The listing builds one solid part. Answer for the finished solid, in the listing's coordinates (mm). Face numbers are marked on the shaded views. A direction names the side the tool comes from. Coordinates: 2 decimals unless noted, no trailing zeros. Order: outer loops, then holes, each group sorted by start corner. A loop starts at its lowest first (then second) coordinate and runs counter-clockwise, first axis right, second up. Notation, with made-up numbers: (-37, 34) -> (-25, 34) arc R14 ccw to (-25, 52) -> close; hole circle Ø11 at (-25.75, 13). An arc over 180 degrees is marked (long way). Answer in a Markdown table with one row per item.
```python
from build123d import *

# Parameters (mm, degrees)
BASPROSKE_W         = 40
BASPROSKE_H         = 25
TOOTHCUT_DEPTH      = 54.38539126
TEETHCUTS_COUNT     = 23
TEETHCUTS_ANGLE     = 344.347826087
BORSKE_R            = 0.4
BORE_DEPTH          = 50.0000508
CUT_EXTRUDE_1_DEPTH = 54.3731118
SKETCH_2_R          = 1.6
CUT_EXTRUDE_2_DEPTH = 54.3731118
EXTRUDE_1_DEPTH     = 40
SKETCH_5_R          = 1.6
CUT_EXTRUDE_3_DEPTH = 61.166132826
CUT_EXTRUDE_4_DEPTH = 61.571969914
SKETCH_7_W          = 12
SKETCH_7_H          = 22
CUT_EXTRUDE_5_DEPTH = 61.166132826
SKETCH_8_R          = 2.6
CUT_EXTRUDE_6_DEPTH = 61.571969914
SKETCH_10_R         = 1.6
SKETCH_10_W         = 12
SKETCH_10_H         = 22
CUT_EXTRUDE_7_DEPTH = 61.166132826
CUT_EXTRUDE_9_DEPTH = 60.774271549


with BuildPart() as part:
    # BasProSke → Base-Revolve (revolve)
    with BuildSketch(Plane(origin=(0, 0, 0), x_dir=(1, 0, 0), z_dir=(0, 1, 0)), mode=Mode.PRIVATE) as base_revolve_sk:
        with Locations((20, 12.5)):
            Rectangle(BASPROSKE_W, BASPROSKE_H)
    revolve(base_revolve_sk.sketch.rotate(Axis((-10, 0, 0), (1, 0, 0)), 180), axis=Axis((-10, 0, 0), (1, 0, 0)))

    # TooCutSke → ToothCut (cut, through all)
    with BuildSketch(Plane(origin=(0, 0, 0), x_dir=(0, 0, -1), z_dir=(1, 0, 0))):
        with BuildLine():
            ThreePointArc((0.960248578, 20.47649686), (0, 20.499), (-0.960248578, 20.47649686))
            ThreePointArc((-0.960248578, 20.47649686), (-1.62297083, 22.794554384), (-2.865164893, 24.860842208))
            ThreePointArc((-2.865164893, 24.860842208), (0, 25.0254), (2.865164893, 24.860842208))
            ThreePointArc((2.865164893, 24.860842208), (1.62297083, 22.794554384), (0.960248578, 20.47649686))
        make_face()
    toothcut = extrude(amount=TOOTHCUT_DEPTH, mode=Mode.SUBTRACT)

    # TeethCuts: ToothCut ×23 about axis
    teethcuts_axis = Axis((-10, 0, 0), (1, 0, 0))
    for i in range(1, TEETHCUTS_COUNT):
        add(toothcut.rotate(teethcuts_axis, i * TEETHCUTS_ANGLE / (TEETHCUTS_COUNT - 1)), mode=Mode.SUBTRACT)

    # BorSke → Bore (cut, symmetric)
    with BuildSketch(Plane(origin=(0, 0, 0), x_dir=(0, 0, -1), z_dir=(1, 0, 0))):
        with Locations(Location((0, 0, 0), (0, 0, 180))):
            Circle(BORSKE_R)
    extrude(amount=BORE_DEPTH, both=True, mode=Mode.SUBTRACT)

    # 草图1 → 切除-拉伸1 (cut, through all)
    with BuildSketch(Plane(origin=(40, 0, 0), x_dir=(0, 0, -1), z_dir=(1, 0, 0))):
        Polygon((0, 0), (0, -25), (-13.134994366, -31.325673685), (-39.860156169, 4.307875386), (-10.07883231, 32.723680029), (33.144547114, 17.371523179), (23.556523053, 8.371990304), align=None)
    extrude(amount=-CUT_EXTRUDE_1_DEPTH, mode=Mode.SUBTRACT)

    # 草图2 → 切除-拉伸2 (cut, through all)
    with BuildSketch(Plane.ZY):
        Circle(SKETCH_2_R)
    extrude(amount=-CUT_EXTRUDE_2_DEPTH, mode=Mode.SUBTRACT)

    # 草图4 → 凸台-拉伸1 (add)
    with BuildSketch(Plane(origin=(40, 0, 0), x_dir=(0, 0, -1), z_dir=(1, 0, 0))):
        with BuildLine():
            Line((0, -4), (0, -11))
            ThreePointArc((0, -11), (-2.636038969, -4.636038969), (-9, -2))
            Line((-9, -2), (-37.99952025, -2))
            Line((-37.99952025, -2), (-37.99952025, 4))
            Line((-37.99952025, 4), (23.556523053, 8.371990304))
            Line((23.556523053, 8.371990304), (1.507617475, 0.535807379))
            ThreePointArc((1.507617475, 0.535807379), (-1.307151829, 0.922688515), (0, -1.6))
            Line((0, -1.6), (0, -4))
        make_face()
    extrude(amount=-EXTRUDE_1_DEPTH)

    # 草图5 → 切除-拉伸3 (cut, through all)
    with BuildSketch(Plane.XZ.offset(1)):
        with Locations(Location((30, 15.99952025, 0), (0, 0, 270))):
            Circle(SKETCH_5_R)
        with Locations(Location((30, 32.99952025, 0), (0, 0, 270))):
            Circle(SKETCH_5_R)
        with Locations(Location((10, 32.99952025, 0), (0, 0, 90))):
            Circle(SKETCH_5_R)
        with Locations(Location((10, 15.99952025, 0), (0, 0, 90))):
            Circle(SKETCH_5_R)
    extrude(amount=-CUT_EXTRUDE_3_DEPTH, mode=Mode.SUBTRACT)

    # 草图6 → 切除-拉伸4 (cut, through all)
    with BuildSketch(Plane.ZY):
        with BuildLine():
            Line((-6.882467579, 1.277356656), (-16.222959293, 3.010912119))
            ThreePointArc((-16.222959293, 3.010912119), (-13.76317845, -9.100819686), (-3.581631723, -16.106579842))
            Line((-3.581631723, -16.106579842), (-3.581631723, -6.014309121))
            ThreePointArc((-3.581631723, -6.014309121), (-6.377024463, -2.886790432), (-6.882467579, 1.277356656))
        make_face()
    extrude(amount=-CUT_EXTRUDE_4_DEPTH, mode=Mode.SUBTRACT)

    # 草图7 → 切除-拉伸5 (cut, through all)
    with BuildSketch(Plane.XZ.offset(1)):
        with Locations((20, 21.99952025)):
            Rectangle(SKETCH_7_W, SKETCH_7_H)
    extrude(amount=-CUT_EXTRUDE_5_DEPTH, mode=Mode.SUBTRACT)

    # 草图8 → 切除-拉伸6 (cut, through all)
    with BuildSketch(Plane(origin=(40, 0, 0), x_dir=(0, 0, -1), z_dir=(1, 0, 0))):
        Circle(SKETCH_8_R)
    extrude(amount=-CUT_EXTRUDE_6_DEPTH, mode=Mode.SUBTRACT)

    # 草图10 → 切除-拉伸7 (cut, through all)
    with BuildSketch(Plane(origin=(0, -1, 0), x_dir=(1, 0, 0), z_dir=(0, 1, 0))):
        with Locations(Location((10, -15.99952025, 0), (0, 0, 90))):
            Circle(SKETCH_10_R)
        with Locations(Location((10, -32.99952025, 0), (0, 0, 90))):
            Circle(SKETCH_10_R)
        with Locations(Location((30, -15.99952025, 0), (0, 0, 90))):
            Circle(SKETCH_10_R)
        with Locations(Location((30, -32.99952025, 0), (0, 0, 90))):
            Circle(SKETCH_10_R)
        with Locations((20, -21.99952025)):
            Rectangle(SKETCH_10_W, SKETCH_10_H)
    extrude(amount=-CUT_EXTRUDE_7_DEPTH, mode=Mode.SUBTRACT)

    # 草图12 → 切除-拉伸9 (cut, through all)
    with BuildSketch(Plane.XZ.offset(2)):
        Polygon((5, 37.99952025), (0, 9), (0, 37.99952025), align=None)
        Polygon((35, 37.99952025), (40, 9), (40, 37.99952025), align=None)
    extrude(amount=-CUT_EXTRUDE_9_DEPTH, mode=Mode.SUBTRACT)


solid = part.part
```
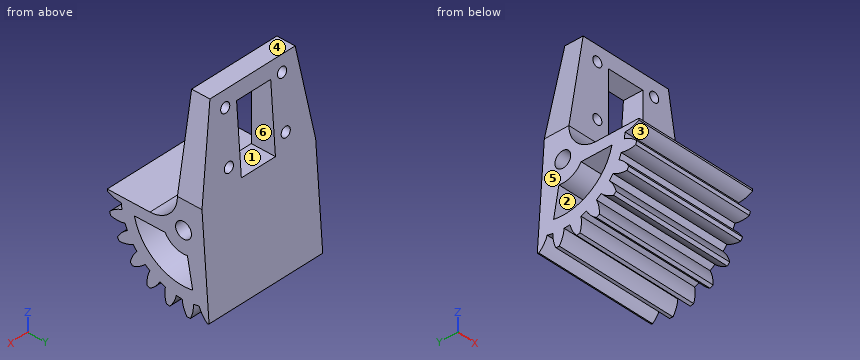
(1) A cutting plane is placed at A-A, the plane x = 22. Count the separate pieces of the cut face and the enclosed holes in it, then the cut area to 3 significant figures.
Check values:
| item | result |
|---|---|
| separate pieces | 2 |
| enclosed holes | 2 |
| area | 527 mm² |
(2) Which of the six approach directions +Z, -Z, +X, -X, +Y, -Y give full straight-line access (tool end or side, diameter ignored) to the marked faces 1, 2 and 3?
Check values:
| item | result |
|---|---|
| face 1 | +Y, -Y |
| face 2 | +X, -X |
| face 3 | +X, -X, -Y |
(3) For a pull along X with two mould halves and no side action, classify the marked faces 4, 5 and 6 as released by +X, released by -X, zero draft, split by the parting line, or undercut.
Check values:
| item | result |
|---|---|
| face 4 | zero draft |
| face 5 | released by -X |
| face 6 | undercut |
(4) Flat-ended cylindrical pins translate along their axes: pin 1 (2.5 mm diameter, centred on x = 30, z = 16, fed in from +Y); pin 2 (5 mm diameter, centred on x = 10, z = 16, fed in from +Y); pin 3 (4 mm diameter, centred on x = 28.5, y = -15, fed in from +Z); pin 4 (5 mm diameter, centred on x = 32.5, y = -16, fed in from -Z). Find the tip coordinate at first contact, or state that the pin passes through.
Check values:
| item | result |
|---|---|
| pin 1 | through |
| pin 2 | y = 5.74 |
| pin 3 | z = 0 |
| pin 4 | z = -18.65 |
(5) A cutting plane is placed at B-B, the plane y = -3.5. Determine the outline of the cut face in (x, z), then the cut area to 3 significant figures.
Check values:
| item | result |
|---|---|
| outline | (0, -23.21) -> (40, -23.21) -> (40, -16.12) -> (0, -16.12) -> close; (0, -6.06) -> (40, -6.06) -> (40, 4.03) -> (0, 4.03) -> close |
| area | 687 mm² |
(6) Find the intervals of material crossed by line 1 along Z through (x, y) = (32.5, -20); line 2 along Z through (x, y) = (30, 1); line 3 along Y through (x, z) = (15, -8), in increasing order. Write a range as from..to.
Check values:
| item | result |
|---|---|
| line 1 | -13.39..-10.3, -7.46..0 |
| line 2 | -24.76..-16.47, -6.93..-2.4, 2.4..14.4, 17.6..31.4, 34.6..38 |
| line 3 | -18.87..-14.43, 1.48..7.27 |
